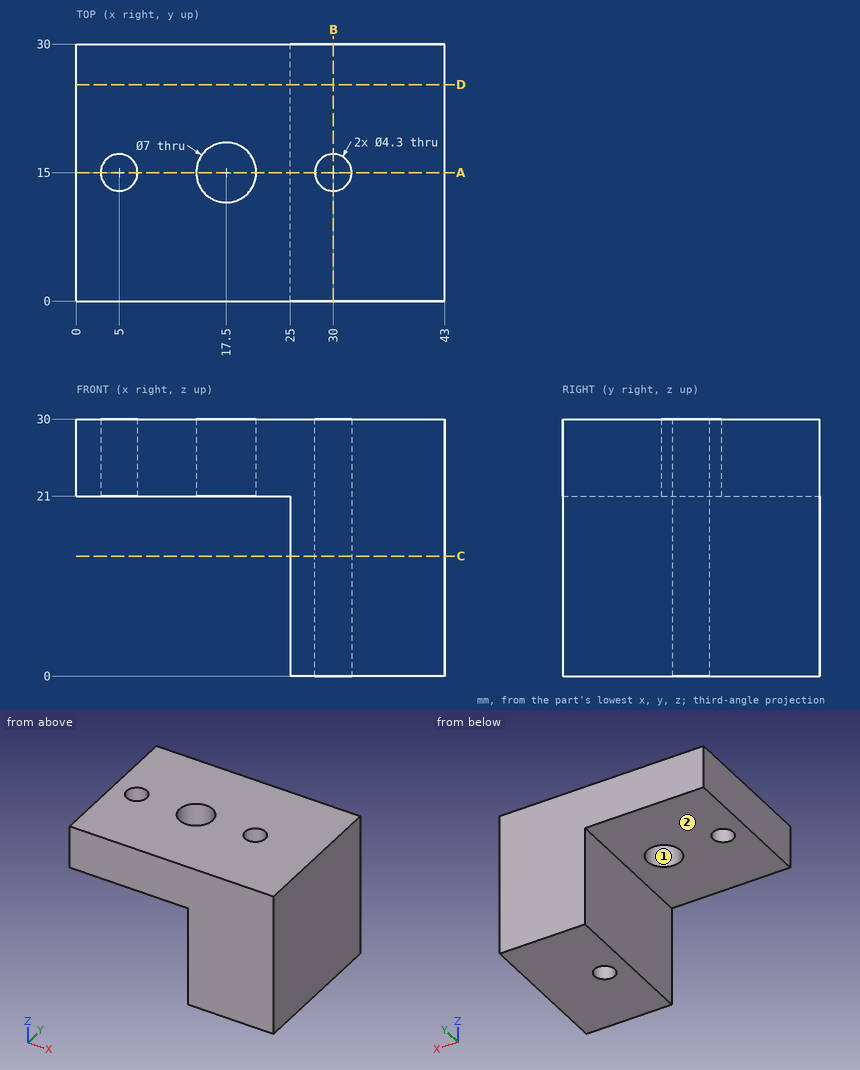
Design review of the part shown in the three views and the two pictorial views. Dimensions are in mm from the part's minimum x, y and z. A direction names the side the tool comes from. Coordinates: 2 decimals unless noted, no trailing zeros. Write each loop counter-clockwise with the first axis right and the second up, starting at its lowest first coordinate (ties: lowest second). Pieces come first, ordered by that corner, then holes.
1) We need section A-A on y = 15. State the section outline as (x, z) points.
2) We need section D-D on y = 25.25. State the section outline as (x, z) points.
3) We need section C-C on z = 14. State the section outline as (x, y) points.
4) Clearance check with flat-ended pins moving along their axes: pin 1 Ø5 at (x, y) = (5, 15) entering from -Z; pin 2 Ø10.5 at (y, z) = (15, 11) entering from -X; pin 3 Ø12 at (x, z) = (23.5, 10) entering from +Y. State where each tip first meets the part, or that it passes through.
5) We need section B-B on x = 30. State the section outline as (y, z) points.
6) To check wall thickness, follow probe 1 along Y at (x, z) = (17.5, 27.25); probe 2 along Y at (x, z) = (5, 25.25); probe 3 along X at (y, z) = (25.5, 9.75). State the ranges of each line that lie inside material, in increasing order.
7) Machinability: for the marked faces 1 and 2, which of the approach directions +Z, -Z, +X, -X, +Y, -Y give a long, thin tool a straight path to every point of the face, cutting with its end or side? Answer none if there is none.
Answer list:
1. outline: (0, 21) - (2.85, 21) - (2.85, 30) - (0, 30) - close; (7.15, 21) - (14, 21) - (14, 30) - (7.15, 30) - close; (21, 21) - (25, 21) - (25, 0) - (27.85, 0) - (27.85, 30) - (21, 30) - close; (32.15, 0) - (43, 0) - (43, 30) - (32.15, 30) - close
2. outline: (0, 21) - (25, 21) - (25, 0) - (43, 0) - (43, 30) - (0, 30) - close
3. outline: (25, 0) - (43, 0) - (43, 30) - (25, 30) - close; hole circle Ø4.3 at (30, 15)
4. pin 1: stops at z = 21
4. pin 2: stops at x = 25
4. pin 3: stops at y = 30
5. outline: (0, 0) - (12.85, 0) - (12.85, 30) - (0, 30) - close; (17.15, 0) - (30, 0) - (30, 30) - (17.15, 30) - close
6. probe 1: y = 0 to 11.5, 18.5 to 30
6. probe 2: y = 0 to 12.85, 17.15 to 30
6. probe 3: x = 25 to 43
7. face 1: +Z, -Z
7. face 2: -Z, -X, +Y, -Y
